Work out the finished part from the listing and answer in its coordinate system (mm). Face numbers are marked on the shaded views. Coordinates: 2 decimals unless noted, no trailing zeros. Order: outer loops, then holes, each group sorted by start corner. A loop starts at its lowest first (then second) coordinate and runs counter-clockwise, first axis right, second up. Notation, with made-up numbers: (85, 3.25) - (114, 3.25) arc R21 cw to (114, 35.25) - close; hole circle Ø3 at (30, 61). An arc over 180 degrees is marked (long way). Answer as a JSON object with one key per item and string values. Group by question number.
1) The mould has two halves that part along Y. Classify the marked faces 1, 2 and 3: released by +Y, released by -Y, zero draft, split by the parting line, or undercut.
2) Each of these flat-tipped pins is pushed along its axis until it touches: P1, Ø1, axis at x = 7, y = -5, coming from the +Z side; P2, Ø2, axis at x = 4.5, y = -5.5, coming from the -Z side; P3, Ø10, axis at y = 0, z = 0, coming from the -X side; P4, Ø1.5, axis at x = 4, z = 2.5, coming from the -Y side. Where does it stop, or does it pass through?
3) Section C-C (x = 3.5) is taken. Give the vertices of the cut face in (y, z), plus the area to 3 significant figures.
4) Find the intervals of material crossed by line 1 along Y through (x, z) = (2, 0); line 2 along Y through (x, z) = (6, 2); line 3 along Z through (x, y) = (4.25, 2.5), in increasing order.
5) Section A-A (y = 0) is taken. Give the vertices of the cut face in (x, z).
6) Section D-D (x = 8.75) is taken. Give the vertices of the cut face in (y, z), plus the area to 3 significant figures.
from build123d import *

# Parameters (mm, degrees)
ESQUISSE1_R             = 11.82
BOSS_EXTRU_1_DEPTH      = 9.4
ESQUISSE2_R             = 6.2
ENL_V_MAT_EXTRU_1_DEPTH = 20.177716235
CONG_3_R                = 2


with BuildPart() as part:
    # Esquisse1 → Boss.-Extru.1 (new body)
    with BuildSketch(Plane(origin=(0, 0, 0), x_dir=(0, 0, -1), z_dir=(1, 0, 0))):
        Circle(ESQUISSE1_R)
    extrude(amount=BOSS_EXTRU_1_DEPTH)

    # Esquisse2 → Enlèv. mat.-Extru.1 (cut, through all)
    with BuildSketch(Plane(origin=(9.4, 0, 0), x_dir=(0, 0, -1), z_dir=(1, 0, 0))):
        Circle(ESQUISSE2_R)
    extrude(amount=-ENL_V_MAT_EXTRU_1_DEPTH, mode=Mode.SUBTRACT)

    # Congé3
    cong_3_edges = [part.edges().sort_by_distance(p)[0] for p in [
        (0, 0, 11.82),
        (9.4, 0, 11.82),
    ]]
    fillet(cong_3_edges, radius=CONG_3_R)


solid = part.part
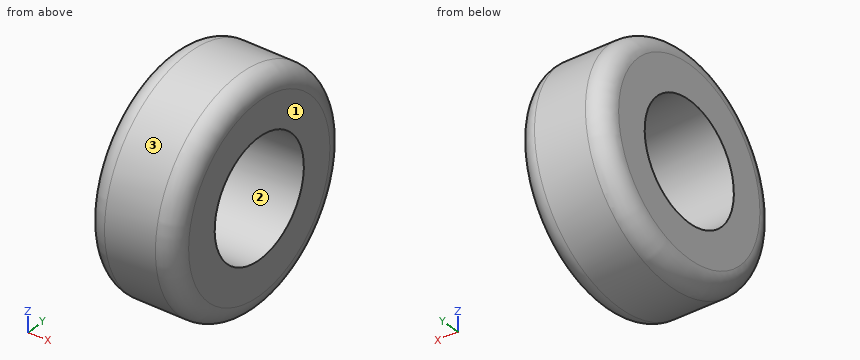
Report:
{
 "1": {"face 1": "zero draft", "face 2": "undercut", "face 3": "split by the parting line"},
 "2": {"P1": "stops at z = 10.93", "P2": "stops at z = -10.93", "P3": "passes through", "P4": "stops at y = -11.69"},
 "3": {"outline": "circle Ø23.64 at (0, 0); hole circle Ø12.4 at (0, 0)", "area": "318 mm²"},
 "4": {"line 1": "y = -11.82 to -6.2, 6.2 to 11.82", "line 2": "y = -11.65 to -5.87, 5.87 to 11.65", "line 3": "z = -11.55 to -5.67, 5.67 to 11.55"},
 "5": {"outline": "(0, -9.82) arc R2 ccw to (2, -11.82) - (7.4, -11.82) arc R2 ccw to (9.4, -9.82) - (9.4, -6.2) - (0, -6.2) - close; (0, 6.2) - (9.4, 6.2) - (9.4, 9.82) arc R2 ccw to (7.4, 11.82) - (2, 11.82) arc R2 ccw to (0, 9.82) - close"},
 "6": {"outline": "circle Ø22.59 at (0, 0); hole circle Ø12.4 at (0, 0)", "area": "280 mm²"}
}
